Read the model definition and answer for the solid it produces. Units are mm, in the model's axes. A direction names the side the tool comes from. Give positions to 0.01 mm unless a question says otherwise; leave off trailing zeros. Loops run counter-clockwise (first coordinate to the right, second up) from the corner with the lowest first, then second, coordinate; pieces in that order, holes last. Notation, with made-up numbers: (34, 47) - (86, 47) arc R20 cw to (86, 79) - close; hole circle Ø4 at (14, 48). An arc over 180 degrees is marked (long way). Use a Markdown table: item, result. Add a question column.
Item 1: A cutting plane is placed at C-C (x = 0). Determine the outline of the cut face in (y, z), plus the area to 4 significant figures.
Item 2: Which of the six approach directions +Z, -Z, +X, -X, +Y, -Y give full straight-line access (tool end or side, diameter ignored) to faces 1 (the face through (-11, 37, 14)), 2 (the face through (11, 37, 15)), 3 (the face through (0.98, 33.11, 4.93)), 4 (the face through (7, 37, 13))?
Item 3: A cutting plane is placed at B-B (z = -36.77). Determine the outline of the cut face in (x, y).
Item 4: Consider probe 1 along X at (y, z) = (35.5, 15.5); probe 2 along Z at (x, y) = (-2.5, 10); probe 3 along X at (y, z) = (71.5, -45). Determine where each line is inside the solid, lowest interval first. Write a range as [from, to].
Item 5: A cutting plane is placed at D-D (y = 37.5). Give the number of separate pieces and of enclosed holes in the cut face, plus the area to 3 significant figures.
Item 6: For a pull along X with two mould halves and no side action, classify faces 5 (the face through (-78, 37, 8.5)), 6 (the face through (1, 74, 2)), 7 (the face through (78, 37, 8.5)), 8 (the face through (-76, 37, -50)) as +X half, -X half, draft (parallel to the pull), parting line (faces both ways), or undercut.
Item 7: A cutting plane is placed at A-A (y = 21.5). Determine the outline of the cut face in (x, z).
Item 8: Each of these flat-tipped pins is pushed along its axis until it touches: P1, Ø7, axis at y = 47, z = 14, coming from the -X side; P2, Ø1, axis at x = -49.5, y = 44.5, coming from the +Z side; P3, Ø3, axis at y = 45.5, z = 13.5, coming from the +X side; P4, Ø2, axis at y = 45.5, z = 7.5, coming from the +X side. Where does it stop, or does it pass through?
from build123d import *

# Parameters (mm, degrees)
SKETCH1_W               = 14
SKETCH1_H               = 6
BOSS_EXTRUDE1_DEPTH     = 75
SKETCH2_R               = 4.5
CUT_EXTRUDE1_DEPTH      = 16
CUT_EXTRUDE2_DEPTH      = 177.287407378
CUT_EXTRUDE2_DEPTH_BACK = 177.287407378
SKETCH3_R               = 4.5
CHAMFER1_SIZE           = 3
SKETCH4_R               = 4
CUT_EXTRUDE3_DEPTH      = 183.773083357


with BuildPart() as part:
    # Sketch1 → Boss-Extrude1 (new body)
    with BuildSketch(Plane(origin=(0, 0, 0), x_dir=(1, 0, 0), z_dir=(0, 1, 0))):
        Polygon((72, 0), (-72, 0), (-72, 50), (-79.5, 50), (-79.5, -10), (-11, -10), (-11, -19), (11, -19), (11, -10), (79.5, -10), (79.5, 50), (72, 50), align=None)
        with Locations((0, -13)):
            Rectangle(SKETCH1_W, SKETCH1_H, mode=Mode.SUBTRACT)
    extrude(amount=BOSS_EXTRUDE1_DEPTH)

    # Sketch2 → Cut-Extrude1 (cut)
    with BuildSketch(Plane(origin=(0, 0, 0), x_dir=(-1, 0, 0), z_dir=(0, 0, -1))):
        with Locations((0, 37.5)):
            Circle(SKETCH2_R)
    extrude(amount=-CUT_EXTRUDE1_DEPTH, mode=Mode.SUBTRACT)

    # Sketch3 → Cut-Extrude2 (cut, two sides: drawn at the far end of the back side and taken through both)
    with BuildSketch(Plane(origin=(-72, 0, 0), x_dir=(0, 0, -1), z_dir=(1, 0, 0)).offset(-CUT_EXTRUDE2_DEPTH_BACK)):
        with Locations((20.77, 37.5)):
            Circle(SKETCH3_R)
    extrude(amount=CUT_EXTRUDE2_DEPTH + CUT_EXTRUDE2_DEPTH_BACK, mode=Mode.SUBTRACT)

    # Chamfer1
    chamfer1_edges = [part.edges().sort_by_distance(p)[0] for p in [
        (79.5, 37.5, 10),
        (-79.5, 37.5, 10),
        (0, 75, 0),
    ]]
    chamfer(chamfer1_edges, length=CHAMFER1_SIZE)

    # Sketch4 → Cut-Extrude3 (cut, through all)
    with BuildSketch(Plane(origin=(79.5, 0, 0), x_dir=(0, 0, -1), z_dir=(1, 0, 0))):
        with Locations((36.77, 21.5)):
            Circle(SKETCH4_R)
    extrude(amount=-CUT_EXTRUDE3_DEPTH, mode=Mode.SUBTRACT)


solid = part.part
Geometry says:
| question | item | result |
|---|---|---|
| 1 | outline | (0, 0) - (33, 0) - (33, 10) - (0, 10) - close; (0, 16) - (75, 16) - (75, 19) - (0, 19) - close; (42, 0) - (72, 0) - (75, 3) - (75, 10) - (42, 10) - close |
| 1 | area | 880.5 mm² |
| 2 | face 1 | +Z, -X, +Y, -Y |
| 2 | face 2 | +Z, +X, +Y, -Y |
| 2 | face 3 | -Z |
| 2 | face 4 | +Y, -Y |
| 3 | outline | (-79.5, 0) - (-72, 0) - (-72, 17.5) - (-79.5, 17.5) - close; (-79.5, 25.5) - (-72, 25.5) - (-72, 75) - (-79.5, 75) - close; (72, 0) - (79.5, 0) - (79.5, 17.5) - (72, 17.5) - close; (72, 25.5) - (79.5, 25.5) - (79.5, 75) - (72, 75) - close |
| 4 | probe 1 | [-11, -7], [7, 11] |
| 4 | probe 2 | [0, 10], [16, 19] |
| 4 | probe 3 | [-79.5, -72], [72, 79.5] |
| 5 | separate pieces | 3 |
| 5 | enclosed holes | 0 |
| 5 | area | 2,220 mm² |
| 6 | face 5 | -X half |
| 6 | face 6 | undercut |
| 6 | face 7 | +X half |
| 6 | face 8 | draft |
| 7 | outline | (-79.5, -50) - (-72, -50) - (-72, -40.77) - (-79.5, -40.77) - close; (-79.5, -32.77) - (-72, -32.77) - (-72, 0) - (72, 0) - (72, -32.77) - (79.5, -32.77) - (79.5, 7) - (76.5, 10) - (11, 10) - (11, 19) - (-11, 19) - (-11, 10) - (-76.5, 10) - (-79.5, 7) - close; (72, -50) - (79.5, -50) - (79.5, -40.77) - (72, -40.77) - close; hole (-7, 10) - (7, 10) - (7, 16) - (-7, 16) - close |
| 8 | P1 | x = -11 |
| 8 | P2 | z = 10 |
| 8 | P3 | x = 11 |
| 8 | P4 | x = 79.5 |
